CAD build for the part. Positions are in the model's coordinates, mm. A direction names the side the tool comes from. Give positions to 0.01 mm unless a question says otherwise; leave off trailing zeros. Write each loop counter-clockwise with the first axis right and the second up, starting at its lowest first coordinate (ties: lowest second). Pieces come first, ordered by that corner, then holes. Notation, with made-up numbers: (-37, 82) -> (-19, 82) arc R22 ccw to (-19, 100) -> close; hole circle Ø5 at (-13.5, 75). An arc over 180 degrees is marked (long way). Answer in a Markdown table with one row per item. Add a question column.
```python
from build123d import *

# Parameters (mm, degrees)
HEX_2_DEPTH = 9.525


# Read off the part's stored shape, not the designer's step: ThreadSchematic
with BuildPart() as part:
    # ThreadSchematic outline → ThreadSchematic (revolve)
    with BuildSketch(Plane.YX):
        with BuildLine():
            Line((0, 79.375), (0, 0))
            Line((0, 0), (14.1732, 0))
            Line((14.1732, 0), (16.6624, 2.4892))
            Line((16.6624, 2.4892), (16.6624, 15.875))
            Line((16.6624, 15.875), (13.4239, 15.875))
            ThreePointArc((13.4239, 15.875), (12.70547951, 16.17257951), (12.4079, 16.891))
            Line((12.4079, 16.891), (12.4079, 18.7833))
            Line((12.4079, 18.7833), (12.6746, 19.05))
            Line((12.6746, 19.05), (12.6746, 53.975))
            Line((12.6746, 53.975), (9.144, 53.975))
            ThreePointArc((9.144, 53.975), (8.210053363, 54.361853363), (7.8232, 55.2958))
            Line((7.8232, 55.2958), (7.8232, 59.055))
            Line((7.8232, 59.055), (9.525, 60.7568))
            Line((9.525, 60.7568), (9.525, 77.86243))
            Line((9.525, 77.86243), (8.01243, 79.375))
            Line((8.01243, 79.375), (0, 79.375))
        make_face()
    revolve(axis=Axis((0, 0, 0), (1, 0, 0)))

    # Sketch2 → PreBroach (revolve, cut)
    with BuildSketch(Plane.XY, mode=Mode.PRIVATE) as prebroach_sk:
        Polygon((0, 6.35), (9.525, 6.35), (13.191174209, 0), (0, 0), align=None)
    revolve(prebroach_sk.sketch.rotate(Axis((0, 0, 0), (1, 0, 0)), 90), axis=Axis((0, 0, 0), (1, 0, 0)), mode=Mode.SUBTRACT)

    # Sketch3 → Hex 2 (cut)
    with BuildSketch(Plane.ZY):
        Polygon((-6.35, -3.666174209), (-6.35, 3.666174209), (0, 7.332348419), (6.35, 3.666174209), (6.35, -3.666174209), (0, -7.332348419), align=None)
    extrude(amount=-HEX_2_DEPTH, mode=Mode.SUBTRACT)


solid = part.part
```
Item 1: Mould opens along X. For faces 1 (the face through (0, 0.2, 6.5)), 2 (the face through (9.276, 15.893, 5.005)), 3 (the face through (17.85, 11.835, 3.727)) say: released by +X, released by -X, zero draft, split by the parting line, or undercut.
Item 2: Probe L1, parallel to X at y = -9, z = -5 (3 decimals); L2, parallel to X at y = 7.5, z = -4; L3, parallel to X at y = 6, z = 12.5 (3 decimals). List the from-to ranges inside material, lowest first. Write a range as from..to.
Item 3: Drop flat-ended pins along their axis: pin 1 Ø1 at (y, z) = (-4, -0.5) entering from -X; pin 2 Ø12 at (y, z) = (-11.5, -12.5) entering from +X (3 decimals); pin 3 Ø2 at (x, y) = (56.5, -2.5) entering from +Z. Give the stop position or say it passes through.
Item 4: Slice it at C-C, the plane x = 71. List the corners of the cut face in (y, z) (3 decimals).
Item 5: Slice it at B-B, the plane x = 29.5. List the corners of the cut face in (y, z).
Item 6: Which spindle directions (+Z, -Z, +X, -X, +Y, -Y) get a long thin tool onto all of the face, cutting with end or side? Do faces 4 (the face through (53.975, 7, 7)), 5 (the face through (79.375, 0, 0)), 6 (the face through (4.696, 5.474, -3.219)), 7 (the face through (15.875, 1, 14)). Say none if no direction does.
Item 7: Slice it at A-A, the plane x = 7. List the corners of the cut face in (y, z).
Answer key:
| question | item | result |
|---|---|---|
| 1 | face 1 | released by -X |
| 1 | face 2 | zero draft |
| 1 | face 3 | undercut |
| 2 | L1 | x = 0..53.975 |
| 2 | L2 | x = 0..54.14, 59.73..78.89 |
| 2 | L3 | x = 0..15.875 |
| 3 | pin 1 | stops at x = 10.58 |
| 3 | pin 2 | stops at x = 53.975 |
| 3 | pin 3 | stops at z = 7.68 |
| 4 | outline | circle Ø19.05 at (0, 0) |
| 5 | outline | circle Ø25.35 at (0, 0) |
| 6 | face 4 | none |
| 6 | face 5 | +Z, -Z, +X, +Y, -Y |
| 6 | face 6 | -X |
| 6 | face 7 | +X |
| 7 | outline | circle Ø33.32 at (0, 0); hole (-7.33, 0) -> (-3.67, -6.35) -> (3.67, -6.35) -> (7.33, 0) -> (3.67, 6.35) -> (-3.67, 6.35) -> close |
